from build123d import *

# Parameters (mm, degrees)
CUT_EXTRUDE2_DEPTH      = 974.845833675
CUT_EXTRUDE2_DEPTH_BACK = 974.845833675
SKETCH4_R               = 5
BOSS_EXTRUDE1_REACH     = 967.407
SKETCH10_R              = 10
SKETCH10_R_2            = 7
CHAMFER1_SIZE           = 1.5
SKETCH24_R              = 15
SKETCH24_R_2            = 10
BOSS_EXTRUDE2_DEPTH     = 265
CHAMFER2_SIZE           = 2.044647147
MIRROR1_START           = -525
MIRROR1_OUTLINE_R       = 10
MIRROR1_DEPTH           = 265


with BuildPart() as part:
    # Sweep-Thin1: sweep along a path in Sketch1
    with BuildLine(Plane(origin=(0, 0, 0), x_dir=(1, 0, 0), z_dir=(0, 1, 0))) as sweep_thin1_path:
        Line((0, 0), (0, 810))
        ThreePointArc((0, 810), (11.715728753, 838.284271247), (40, 850))
        Line((40, 850), (380, 850))
        ThreePointArc((380, 850), (408.284271247, 838.284271247), (420, 810))
        Line((420, 810), (420, 0))
    # Sketch3 → Sweep-Thin1 (sweep)
    with BuildSketch(Plane.XY):
        with BuildLine():
            Line((14.05, 19.05), (-14.05, 19.05))
            ThreePointArc((-14.05, 19.05), (-17.585533906, 17.585533906), (-19.05, 14.05))
            Line((-19.05, 14.05), (-19.05, -14.05))
            ThreePointArc((-19.05, -14.05), (-17.585533906, -17.585533906), (-14.05, -19.05))
            Line((-14.05, -19.05), (14.05, -19.05))
            ThreePointArc((14.05, -19.05), (17.585533906, -17.585533906), (19.05, -14.05))
            Line((19.05, -14.05), (19.05, 14.05))
            ThreePointArc((19.05, 14.05), (17.585533906, 17.585533906), (14.05, 19.05))
        make_face()
        with BuildLine():
            Line((14.05, 15.875), (-14.05, 15.875))
            ThreePointArc((-14.05, 15.875), (-15.340469876, 15.340469876), (-15.875, 14.05))
            Line((-15.875, 14.05), (-15.875, -14.05))
            ThreePointArc((-15.875, -14.05), (-15.340469876, -15.340469876), (-14.05, -15.875))
            Line((-14.05, -15.875), (14.05, -15.875))
            ThreePointArc((14.05, -15.875), (15.340469876, -15.340469876), (15.875, -14.05))
            Line((15.875, -14.05), (15.875, 14.05))
            ThreePointArc((15.875, 14.05), (15.340469876, 15.340469876), (14.05, 15.875))
        make_face(mode=Mode.SUBTRACT)
    sweep(path=sweep_thin1_path.line)

    # Sketch4 → Cut-Extrude2 (cut, two sides: drawn at the far end of the back side and taken through both)
    with BuildSketch(Plane(origin=(0, 0, 0), x_dir=(0, 0, -1), z_dir=(1, 0, 0)).offset(-CUT_EXTRUDE2_DEPTH_BACK)):
        with Locations((30, 0)):
            Circle(SKETCH4_R)
        with Locations((80, 0)):
            Circle(SKETCH4_R)
        with Locations((180.955115779, 0)):
            Circle(SKETCH4_R)
    extrude(amount=CUT_EXTRUDE2_DEPTH + CUT_EXTRUDE2_DEPTH_BACK, mode=Mode.SUBTRACT)

    # Sketch10 → Boss-Extrude1 (add, up to next)
    with BuildSketch(Plane.ZY.offset(-400.95), mode=Mode.PRIVATE) as boss_extrude1_sk1:
        with Locations(Location((-560, 0, 0), (0, 0, 180))):
            Circle(SKETCH10_R)
        with Locations(Location((-560, 0, 0), (0, 0, 180))):
            Circle(SKETCH10_R_2, mode=Mode.SUBTRACT)
    boss_extrude1_tool1 = extrude(boss_extrude1_sk1.sketch, amount=BOSS_EXTRUDE1_REACH, mode=Mode.PRIVATE) - part.part
    # Sketch10 → Boss-Extrude1 (add, up to next)
    with BuildSketch(Plane.ZY.offset(-400.95), mode=Mode.PRIVATE) as boss_extrude1_sk2:
        with Locations(Location((-260, 0, 0), (0, 0, 180))):
            Circle(SKETCH10_R)
        with Locations(Location((-260, 0, 0), (0, 0, 180))):
            Circle(SKETCH10_R_2, mode=Mode.SUBTRACT)
    boss_extrude1_tool2 = extrude(boss_extrude1_sk2.sketch, amount=BOSS_EXTRUDE1_REACH, mode=Mode.PRIVATE) - part.part
    add(boss_extrude1_tool1.solids().sort_by_distance((400.95, 0, -550.282843))[0])
    add(boss_extrude1_tool2.solids().sort_by_distance((400.95, 0, -250.282843))[0])

    # Chamfer1
    chamfer1_edges = [part.edges().sort_by_distance(p)[0] for p in [
        (400.95, 0, -550),
        (19.05, 0, -550),
        (400.95, 0, -250),
        (19.05, 0, -250),
    ]]
    chamfer(chamfer1_edges, length=CHAMFER1_SIZE)

    # Sketch24 → Boss-Extrude2 (add)
    with BuildSketch(Plane.XY.offset(-260)):
        with Locations((420, -33.55)):
            Circle(SKETCH24_R)
        with Locations((420, -33.55)):
            Circle(SKETCH24_R_2, mode=Mode.SUBTRACT)
    extrude(amount=-BOSS_EXTRUDE2_DEPTH)

    # Chamfer2
    # the kernel refuses this chamfer: 2.5, 2.044647147 mm, written as the material it adds along each edge
    with BuildSketch(Plane(origin=(423.840572874, -19.05, -525), x_dir=(1, 0, 0), z_dir=(0, 0, 1))) as chamfer2_piece_1:
        with BuildLine():
            Line((CHAMFER2_SIZE, 0), (2.598026583, -0.952142714))
            ThreePointArc((2.598026583, -0.952142714), (1.357346607, -0.429405376), (0, 0))
            Line((0, 0), (CHAMFER2_SIZE, 0))
        make_face()
    extrude(amount=265)
    with BuildSketch(Plane(origin=(416.159427126, -19.05, -525), x_dir=(-1, 0, 0), z_dir=(0, 0, 1))) as chamfer2_piece_2:
        with BuildLine():
            Line((CHAMFER2_SIZE, 0), (2.598026583, 0.952142714))
            ThreePointArc((2.598026583, 0.952142714), (1.357346607, 0.429405376), (0, 0))
            Line((0, 0), (CHAMFER2_SIZE, 0))
        make_face()
    extrude(amount=265)

    # Mirror1: read off the stored shape, not the designer's step
    # Mirror1 outline → Mirror1 (add)
    with BuildSketch(Plane.XY.offset(MIRROR1_START)):
        with BuildLine():
            Line((-6.340572874, -19.05), (-8.440985911, -21.150413037))
            ThreePointArc((-8.440985911, -21.150413037), (0, -48.55), (8.440985911, -21.150413037))
            Line((8.440985911, -21.150413037), (6.340572874, -19.05))
            Line((6.340572874, -19.05), (-6.340572874, -19.05))
        make_face()
        with Locations((0, -33.55)):
            Circle(MIRROR1_OUTLINE_R, mode=Mode.SUBTRACT)
    extrude(amount=MIRROR1_DEPTH)


solid = part.part
Input: part model. Units: mm. Frame: model coordinates. A direction names the side the tool comes from. Coordinates: 2 decimals unless noted, no trailing zeros. Loops run counter-clockwise (first coordinate to the right, second up) from the corner with the lowest first, then second, coordinate; pieces in that order, holes last.
(1) Section B-B on y = -33.55. Return the cut outline in (x, z).
(2) Pull-direction query (Y, two-part tool) for faces 6 (the face through (404.125, 0, -399)), 7 (the face through (212, 0, -869.05)), 8 (the face through (10, 15.875, -498)); classes: released by +Y, released by -Y, zero draft, split by the parting line, or undercut.
(3) Section A-A on x = 61.5. Return the cut outline in (y, z) (3 decimals).
(4) First-contact query: pin 1 Ø3 at (y, z) = (-41.5, -374) entering from +X; pin 2 Ø5 at (x, y) = (48, -15.5) entering from +Z; pin 3 Ø12 at (x, y) = (206.5, 3) entering from +Z. Flat tips, straight axial feed; report the tip coordinate or a pass-through.
(5) Section C-C on z = -640. Count the separate pieces of the cut face and the enclosed holes in it, then the cut area to 3 significant figures.
(6) Material intervals for probe 1 along X at (y, z) = (-10, -769) (3 decimals); probe 2 along Z at (x, y) = (401, 0) (3 decimals), sorted ascending.
(7) Set-up query: faces 1 (the face through (15.875, 0, -411)), 2 (the face through (-19.05, 0, -411)), 3 (the face through (394.65, 0.197, -824.976)), 4 (the face through (212, 0, -865.875)), 5 (the face through (430.2, -34, -260)). Return all of +Z, -Z, +X, -X, +Y, -Y with unobstructed straight access to the full face (end or side cutting, diameter ignored); none if empty.
Data:
1. outline: (-15, -525) - (-10, -525) - (-10, -260) - (-15, -260) - close; (10, -525) - (15, -525) - (15, -260) - (10, -260) - close; (405, -525) - (410, -525) - (410, -260) - (405, -260) - close; (430, -525) - (435, -525) - (435, -260) - (430, -260) - close
2. face 6: undercut
2. face 7: zero draft
2. face 8: undercut
3. outline: (-19.05, -864.05) arc R5 ccw to (-14.05, -869.05) - (14.05, -869.05) arc R5 ccw to (19.05, -864.05) - (19.05, -835.95) arc R5 ccw to (14.05, -830.95) - (-14.05, -830.95) arc R5 ccw to (-19.05, -835.95) - close; circle Ø20 at (0, -560); circle Ø20 at (0, -260); hole (-15.875, -864.05) arc R1.825 ccw to (-14.05, -865.875) - (14.05, -865.875) arc R1.825 ccw to (15.875, -864.05) - (15.875, -835.95) arc R1.825 ccw to (14.05, -834.125) - (-14.05, -834.125) arc R1.825 ccw to (-15.875, -835.95) - close; hole circle Ø14 at (0, -560); hole circle Ø14 at (0, -260)
4. pin 1: stops at x = 433.54
4. pin 2: stops at z = -830.95
4. pin 3: stops at z = -250
5. separate pieces: 2
5. enclosed holes: 2
5. area: 850 mm2
6. probe 1: x = -19.05 to -15.875, 15.875 to 19.05, 400.95 to 404.125, 435.875 to 439.05
6. probe 2: z = -865.19 to -861.779, -821.875 to -185.955, -175.955 to -85, -75 to -35, -25 to 0
7. face 1: +Z
7. face 2: +Z, -Z, -X, +Y, -Y
7. face 3: +Y, -Y
7. face 4: none
7. face 5: +Z, +X, -X, -Y
